Model file for the job. Use its own axes, mm. Face numbers are marked on the shaded views. A direction names the side the tool comes from. Give positions to 0.01 mm unless a question says otherwise; leave off trailing zeros. Loops run counter-clockwise (first coordinate to the right, second up) from the corner with the lowest first, then second, coordinate; pieces in that order, holes last. Notation, with made-up numbers: M -24.75,-38 L -20.75,-38 A8 cw -20.75,-32 Z; hole C 25.25,15.25 d5. An arc over 180 degrees is marked long. Answer in a Markdown table with one row per item.
Autodesk Fusion 360 part; units mm, degrees
sketch "Sketch1" plane through (0, 0, 0) normal (1, 0, 0) x (0, 0, -1)
  circle A0 centre (0, 0) radius 4
  line L0 (2, 2) -> (-2, 2)
  line L1 (-2, 2) -> (-2, -2)
  line L2 (-2, -2) -> (2, -2)
  line L3 (2, -2) -> (2, 2)
  line L4 (2, 2) -> (-2, -2) construction
  line L5 (-2, 2) -> (2, -2) construction
  dimension "d1" = 8
  dimension "d2" = 4
  dimension "d3" = 4
extrude "Extrude1" add sketch "Sketch1" along normal blind 2
sketch "Sketch2" plane through (2, 0, 0) normal (1, 0, 0) x (0, 0, -1)
  line L0 (2, 2) -> (2, -2)
  line L1 (2, -2) -> (-2, -2)
  line L2 (-2, -2) -> (-2, 2)
  line L3 (-2, 2) -> (2, 2)
  circle A0 centre (0, 0) radius 4
  circle A1 centre (0, 0) radius 7.5
  dimension "d6" = 15
extrude "Extrude2" add sketch "Sketch2" along normal blind 2 contours L0 L1 L2 L3 | A0 | A1
fillet "Fillet1" radius 1 1 edges at (2, -1.4465, 3.7293)
chamfer "Chamfer1" distance 0.5 angle 45 1 edges at (4, -2.7121, 6.9925)
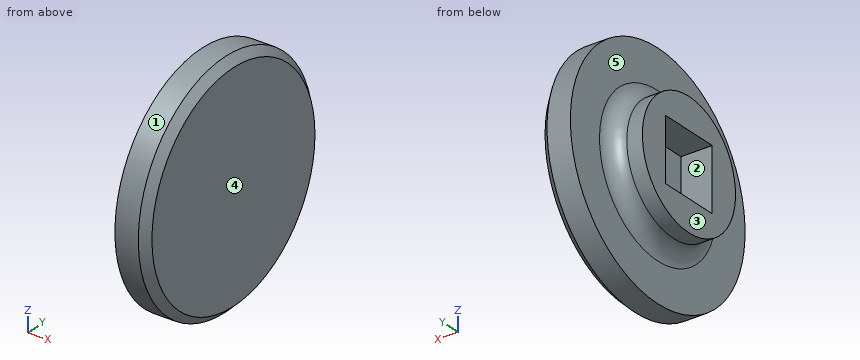
(1) Which spindle directions (+Z, -Z, +X, -X, +Y, -Y) get a long thin tool onto all of the face, cutting with end or side? Do the marked faces 4 and 5. Say none if no direction does.
Established:
| item | result |
|---|---|
| face 4 | +Z, -Z, +X, +Y, -Y |
| face 5 | -X |
(2) Wall check: L1, parallel to X at y = 6, z = 3; L2, parallel to Y at x = 0.4, z = -0.75; L3, parallel to Y at x = 3.15, z = 1.5. Give the ranges that are in metal, low to high.
Established:
| item | result |
|---|---|
| L1 | x = 2 to 4 |
| L2 | y = -3.93 to -2, 2 to 3.93 |
| L3 | y = -7.35 to 7.35 |
(3) Saw through at A-A, the plane z = 0. Give the cut face in (x, y), and give its area (3 significant figures).
Established:
| item | result |
|---|---|
| outline | M 0,-4 L 1,-4 A1 cw 2,-5 L 2,-7.5 L 3.5,-7.5 L 4,-7 L 4,7 L 3.5,7.5 L 2,7.5 L 2,5 A1 cw 1,4 L 0,4 L 0,2 L 2,2 L 2,-2 L 0,-2 Z |
| area | 38.2 mm2 |
(4) Saw through at C-C, the plane x = 0.5. Give the cut face in (y, z), and give its area (3 significant figures).
Established:
| item | result |
|---|---|
| outline | C 0,0 d8; hole M -2,-2 L 2,-2 L 2,2 L -2,2 Z |
| area | 34.3 mm2 |
(5) Saw through at D-D, the plane x = 2.8. Give the cut face in (y, z).
Established:
| item | result |
|---|---|
| outline | C 0,0 d15 |
(6) Flat gauge pins, fed straight in: P1, Ø1, axis at x = 1, y = -0.5, coming from the -Z side; P2, Ø1.5, axis at x = 2.5, y = 3.5, coming from the -Z side; P3, Ø0.6, axis at x = 0.5, z = -1, coming from the -Y side. Where does each tip first touch, or does it go through?
Established:
| item | result |
|---|---|
| P1 | stops at z = -4.11 |
| P2 | stops at z = -6.98 |
| P3 | stops at y = -3.94 |
(7) Mould opens along Z. For the marked faces 1, 2 and 3 say: pulls with the +Z half, pulls with the -Z half, needs draft (parallel to the pull), parting line crosses it, or undercut.
Established:
| item | result |
|---|---|
| face 1 | parting line crosses it |
| face 2 | undercut |
| face 3 | needs draft |
